from build123d import *

# Parameters (mm, degrees)
F0_W     = 190.5
F0_H     = 133.35
F1_DEPTH = 7
F2_W     = 64
F2_H     = 18.6
F3_DEPTH = 3
F4_R     = 3.5
F5_DEPTH = 25


with BuildPart() as f1:
    # F0 (on Top) → F1 (new body)
    with BuildSketch(Plane.XY):
        Rectangle(F0_W, F0_H)
    extrude(amount=F1_DEPTH)

    # F2 (on face) → F3 (cut)
    with BuildSketch(Plane.XY.offset(7)):
        with Locations((-43.25, 54.875)):
            Rectangle(F2_W, F2_H)
        with Locations((43.25, 54.875)):
            Rectangle(F2_W, F2_H)
        with Locations((43.25, -54.875)):
            Rectangle(F2_W, F2_H)
        with Locations((-43.25, -54.875)):
            Rectangle(F2_W, F2_H)
    extrude(amount=-F3_DEPTH, mode=Mode.SUBTRACT)

    # F4 (on face) → F5 (cut)
    with BuildSketch(Plane.XY.offset(7)):
        with Locations((0, -45.575)):
            Circle(F4_R)
        with Locations((0, 45.575)):
            Circle(F4_R)
    extrude(amount=-F5_DEPTH, mode=Mode.SUBTRACT)


solid = f1.part
The model under review builds one solid part; all positions refer to its coordinate system, in mm. A direction names the side the tool comes from. Round coordinates to 2 decimals unless told otherwise and drop trailing zeros. Loops run counter-clockwise (first coordinate to the right, second up) from the corner with the lowest first, then second, coordinate; pieces in that order, holes last. Notation, with made-up numbers: M 36.5,11.5 L 76.5,11.5 A31 cw 76.5,46.5 Z; hole C 44.25,42.25 d1. An arc over 180 degrees is marked long. Answer as CSV lines item,"result".
1. For faces 1 (the face through (-44, -55, 4)), 2 (the face through (95.25, -1, 3)), list the 3-axis set-ups (+Z, -Z, +X, -X, +Y, -Y) from which the entire face can be reached by the end or side of a thin tool; tool diameter is ignored.
Outcome:
face 1,"+Z"
face 2,"+Z, -Z, +X, +Y, -Y"
2. We need section C-C (x = 69). Give the boundary of the cut face in (y, z) (3 decimals), plus the area to 3 significant figures.
Outcome:
outline,"M -66.675,0 L 66.675,0 L 66.675,7 L 64.175,7 L 64.175,4 L 45.575,4 L 45.575,7 L -45.575,7 L -45.575,4 L -64.175,4 L -64.175,7 L -66.675,7 Z"
area,"822 mm2"
3. Draft analysis for pull direction X (two halves, no side actions). For faces 3 (the face through (-0.76, -48.99, 3.55)), 4 (the face through (-1, 1, 0)), 5 (the face through (-95.25, -1, 3)), state which applies: pulls with the +X half, pulls with the -X half, needs draft (parallel to the pull), parting line crosses it, or undercut.
Outcome:
face 3,"undercut"
face 4,"needs draft"
face 5,"pulls with the -X half"
4. Insertion check: pin 1 Ø5.5 at (x, y) = (45, -56) entering from +Z. The pin has a flat end and moves straight along its axis. Give the tip position at first contact, or say it passes through.
Outcome:
pin 1,"stops at z = 4"
5. We need section A-A (x = 0). Give the boundary of the cut face in (y, z) (3 decimals), plus the area to 3 significant figures.
Outcome:
outline,"M -66.675,0 L -49.075,0 L -49.075,7 L -66.675,7 Z; M -42.075,0 L 42.075,0 L 42.075,7 L -42.075,7 Z; M 49.075,0 L 66.675,0 L 66.675,7 L 49.075,7 Z"
area,"835 mm2"
6. To check wall thickness, follow L1, parallel to Y at x = -60.5, z = 5 (3 decimals); L2, parallel to Y at x = 0, z = 3.25 (3 decimals); L3, parallel to Z at x = 33, y = -53.5. State the ranges of each line that lie inside material, in increasing order. Write a range as [from, to].
Outcome:
L1,"y = [-66.675, -64.175], [-45.575, 45.575], [64.175, 66.675]"
L2,"y = [-66.675, -49.075], [-42.075, 42.075], [49.075, 66.675]"
L3,"z = [0, 4]"
7. We need section B-B (y = -52). Give the boundary of the cut face in (x, z), plus the area to 4 significant figures.
Outcome:
outline,"M -95.25,0 L 95.25,0 L 95.25,7 L 75.25,7 L 75.25,4 L 11.25,4 L 11.25,7 L -11.25,7 L -11.25,4 L -75.25,4 L -75.25,7 L -95.25,7 Z"
area,"949.5 mm2"
